```python
from build123d import *

# Parameters (mm, degrees)
SKETCH1_R           = 7.9375
BOSS_EXTRUDE1_DEPTH = 22.352
SKETCH2_R           = 2.38125
CUT_EXTRUDE1_DEPTH  = 26.012391259
SKETCH3_R           = 2.2225
CUT_EXTRUDE2_DEPTH  = 26.012391259


with BuildPart() as part:
    # Sketch1 → Boss-Extrude1 (new body)
    with BuildSketch(Plane.XY):
        Circle(SKETCH1_R)
    extrude(amount=BOSS_EXTRUDE1_DEPTH)

    # Sketch2 → Cut-Extrude1 (cut, through all)
    with BuildSketch(Plane.XY.offset(22.352)):
        Circle(SKETCH2_R)
    extrude(amount=-CUT_EXTRUDE1_DEPTH, mode=Mode.SUBTRACT)

    # Sketch3 → Cut-Extrude2 (cut, through all)
    with BuildSketch(Plane(origin=(0, 0, 0), x_dir=(1, 0, 0), z_dir=(0, 1, 0))):
        with Locations(Location((0, -4.445, 0), (0, 0, 90))):
            Circle(SKETCH3_R)
        with Locations(Location((0, -17.907, 0), (0, 0, 90))):
            Circle(SKETCH3_R)
    extrude(amount=CUT_EXTRUDE2_DEPTH, mode=Mode.SUBTRACT)


solid = part.part
```
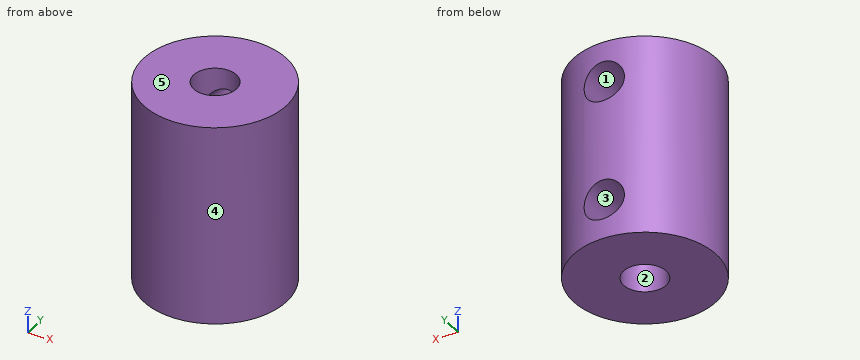
Verification items for the finished model (mm, model axes). Face numbers are marked on the shaded views. A direction names the side the tool comes from. Give positions to 0.01 mm unless a question says otherwise; leave off trailing zeros. Order: outer loops, then holes, each group sorted by start corner. A loop starts at its lowest first (then second) coordinate and runs counter-clockwise, first axis right, second up. Notation, with made-up numbers: M 38,80 L 84,80 A37 ccw 84,117 Z; hole C 80.5,4 d5. An arc over 180 degrees is marked long. Answer in a Markdown table with one row per item. Add a question column.
Item 1: Tool access check on the marked faces 1 and 2. Record the directions out of +Z, -Z, +X, -X, +Y, -Y that give a thin tool (end or side, any length) a straight path to the whole face; none if there is none.
Item 2: Section check D-D, the plane y = 4.25. Enter the section's corners in (x, z) (1 decimal), and give its area (3 significant figures).
Item 3: Section check A-A, the plane x = 0. Enter the section's corners in (y, z).
Item 4: Scan lines: probe 1 along Y at (x, z) = (0, 13); probe 2 along Z at (x, y) = (-1.5, 5); probe 3 along X at (y, z) = (-1.25, 8). Record each from-to range of solid material in increasing order. Write a range as from..to.
Item 5: Gauge pin test, flat ends, axial feed: pin 1 (2 mm diameter, centred on y = 4, z = 5.5, fed in from -X); pin 2 (5 mm diameter, centred on x = -6, z = 16.5, fed in from +Y); pin 3 (1 mm diameter, centred on x = 4, z = 13.5, fed in from -Y). Record the tip position at first contact, or that the pin passes through.
Item 6: Mould release check, pull along X, two halves, no side actions. Record for the marked faces 3, 4 and 5: released by +X, released by -X, zero draft, split by the parting line, or undercut.
Item 7: Section check C-C, the plane z = 7.5. Enter the section's corners in (x, y) (1 decimal).
Item 8: Section check B-B, the plane y = 0. Enter the section's corners in (x, z).
Filled sheet:
| question | item | result |
|---|---|---|
| 1 | face 1 | +Y |
| 1 | face 2 | +Z, -Z |
| 2 | outline | M -6.7,0 L 6.7,0 L 6.7,22.4 L -6.7,22.4 Z; hole C 0,4.4 d4.4; hole C 0,17.9 d4.4 |
| 2 | area | 269 mm^2 |
| 3 | outline | M -7.94,0 L -2.38,0 L -2.38,22.35 L -7.94,22.35 Z; M 2.38,0 L 7.94,0 L 7.94,2.22 L 2.38,2.22 Z; M 2.38,6.67 L 7.94,6.67 L 7.94,15.68 L 2.38,15.68 Z; M 2.38,20.13 L 7.94,20.13 L 7.94,22.35 L 2.38,22.35 Z |
| 4 | probe 1 | y = -7.94..-2.38, 2.38..7.94 |
| 4 | probe 2 | z = 0..2.81, 6.08..16.27, 19.55..22.35 |
| 4 | probe 3 | x = -7.84..-2.03, 2.03..7.84 |
| 5 | pin 1 | stops at x = -7.35 |
| 5 | pin 2 | stops at y = 7.12 |
| 5 | pin 3 | stops at y = -7.12 |
| 6 | face 3 | undercut |
| 6 | face 4 | split by the parting line |
| 6 | face 5 | zero draft |
| 7 | outline | C 0,0 d15.9; hole C 0,0 d4.8 |
| 8 | outline | M -7.94,0 L -2.38,0 L -2.38,22.35 L -7.94,22.35 Z; M 2.38,0 L 7.94,0 L 7.94,22.35 L 2.38,22.35 Z |
